Can you work these out from the drawing? Everything is in mm from the part's minimum corner. Coordinates: 2 decimals unless noted, no trailing zeros. Order: outer loops, then holes, each group sorted by start corner. A loop starts at its lowest first (then second) coordinate and runs counter-clockwise, first axis right, second up. Notation, with made-up numbers: (-22.75, 22.25) - (10.25, 22.25) arc R20 cw to (10.25, 52.25) - close; hole circle Ø8 at (-31, 50). An arc over 180 degrees is marked (long way). Answer as CSV lines item,"result". Start each with the question number.
Item 1: Imagine slicing it at C-C on x = 5. List the corners of the cut face in (y, z) for me.
Item 2: I'm going to push flat-ended pins straight in: pin 1 (9.5 mm diameter, centred on x = 133, y = 90, fed in from -Z); pin 2 (5.5 mm diameter, centred on x = 133, y = 5, fed in from +Z). Where does each tip first touch, or does it pass through?
Item 3: I need wall thicknesses on line 1 (Y direction, x = 133, z = 0.6); line 2 (X direction, y = 38, z = 0.4); line 3 (Y direction, x = 63.5, z = 0.9). Which ranges of each line are inside material? Lowest first, please.
Item 4: Imagine slicing it at D-D on z = 0.55. List the corners of the cut face in (x, y) for me, and give its area (3 significant figures).
Item 5: Imagine slicing it at B-B on x = 133. List the corners of the cut face in (y, z) for me, and give its area (3 significant figures).
Item 6: Imagine slicing it at A-A on y = 48.5. List the corners of the cut face in (x, z) for me, and give its area (3 significant figures).
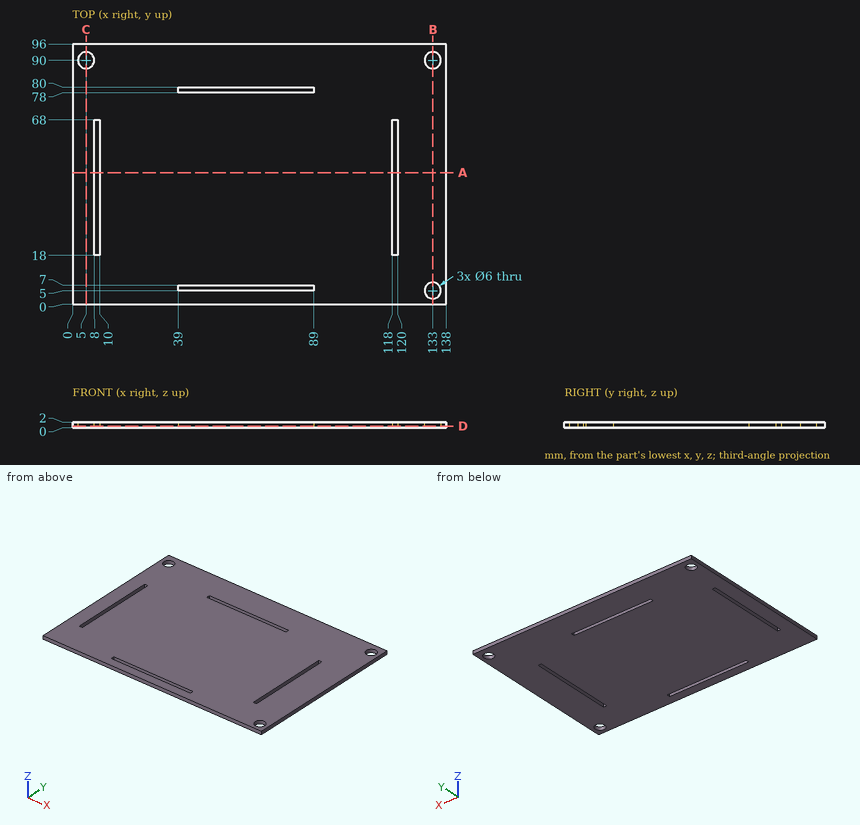
Responses:
1,outline,"(0, 0) - (87, 0) - (87, 2) - (0, 2) - close; (93, 0) - (96, 0) - (96, 2) - (93, 2) - close"
2,pin 1,"stops at z = 0"
2,pin 2,"passes through"
3,line 1,"y = 0 to 2, 8 to 87, 93 to 96"
3,line 2,"x = 0 to 8, 10 to 118, 120 to 138"
3,line 3,"y = 0 to 5, 7 to 78, 80 to 96"
4,outline,"(0, 0) - (138, 0) - (138, 96) - (0, 96) - close; hole circle Ø6 at (5, 90); hole (8, 18) - (10, 18) - (10, 68) - (8, 68) - close; hole (39, 5) - (89, 5) - (89, 7) - (39, 7) - close; hole (39, 78) - (89, 78) - (89, 80) - (39, 80) - close; hole (118, 18) - (120, 18) - (120, 68) - (118, 68) - close; hole circle Ø6 at (133, 5); hole circle Ø6 at (133, 90)"
4,area,"12,800 mm^2"
5,outline,"(0, 0) - (2, 0) - (2, 2) - (0, 2) - close; (8, 0) - (87, 0) - (87, 2) - (8, 2) - close; (93, 0) - (96, 0) - (96, 2) - (93, 2) - close"
5,area,"168 mm^2"
6,outline,"(0, 0) - (8, 0) - (8, 2) - (0, 2) - close; (10, 0) - (118, 0) - (118, 2) - (10, 2) - close; (120, 0) - (138, 0) - (138, 2) - (120, 2) - close"
6,area,"268 mm^2"
